```python
from build123d import *

# Parameters (mm, degrees)
BOSS_EXTRUDE1_DEPTH = 14
SKETCH2_R           = 2.5
SKETCH2_R_2         = 2.25
BOSS_EXTRUDE3_DEPTH = 1.5
SKETCH3_R           = 0.75
BOSS_EXTRUDE4_DEPTH = 8
BOSS_EXTRUDE5_DEPTH = 25.5
SKETCH8_R           = 0.75
BOSS_EXTRUDE7_DEPTH = 1
SKETCH9_R           = 0.75
BOSS_EXTRUDE8_DEPTH = 1


with BuildPart() as part:
    # Sketch1 → Boss-Extrude1 (new body)
    with BuildSketch(Plane.XY):
        with BuildLine():
            Line((1, 0), (23.320898327, 0))
            ThreePointArc((23.320898327, 0), (24.381558498, -0.439339828), (24.820898327, -1.5))
            Line((24.820898327, -1.5), (24.820898327, -11.016992716))
            ThreePointArc((24.820898327, -11.016992716), (24.381558498, -12.077652887), (23.320898327, -12.516992716))
            Line((23.320898327, -12.516992716), (1, -12.516992716))
            ThreePointArc((1, -12.516992716), (0.292893219, -12.224099497), (0, -11.516992716))
            Line((0, -11.516992716), (0, -1))
            ThreePointArc((0, -1), (0.292893219, -0.292893219), (1, 0))
        make_face()
    extrude(amount=BOSS_EXTRUDE1_DEPTH)

    # Sketch2 → Boss-Extrude3 (add)
    with BuildSketch(Plane(origin=(0, 0, 0), x_dir=(0, 0, -1), z_dir=(1, 0, 0))):
        with Locations((-7.367821443, -5.872283843)):
            Circle(SKETCH2_R)
        with Locations((-7.367821443, -5.872283843)):
            Circle(SKETCH2_R_2, mode=Mode.SUBTRACT)
    extrude(amount=-BOSS_EXTRUDE3_DEPTH)

    # Sketch3 → Boss-Extrude4 (add)
    with BuildSketch(Plane.ZY):
        with Locations(Location((7.367821443, -5.872283843, 0), (0, 0, 180))):
            Circle(SKETCH3_R)
    extrude(amount=BOSS_EXTRUDE4_DEPTH)

    # Sketch7 → Boss-Extrude5 (add)
    with BuildSketch(Plane(origin=(0, 0, 0), x_dir=(0, 0, -1), z_dir=(1, 0, 0))):
        with BuildLine():
            Line((-11.394447379, -3.62022901), (-3.393359944, -3.62022901))
            ThreePointArc((-3.393359944, -3.62022901), (-7.393903662, -9.38997212), (-11.394447379, -3.62022901))
        make_face()
    extrude(amount=BOSS_EXTRUDE5_DEPTH)

    # Sketch8 → Boss-Extrude7 (add)
    with BuildSketch(Plane(origin=(25.5, 0, 0), x_dir=(0, 0, -1), z_dir=(1, 0, 0))):
        with Locations((-7.348346706, -5.904616391)):
            Circle(SKETCH8_R)
    extrude(amount=-BOSS_EXTRUDE7_DEPTH)

    # Sketch9 → Boss-Extrude8 (add)
    with BuildSketch(Plane(origin=(25.5, 0, 0), x_dir=(0, 0, -1), z_dir=(1, 0, 0))):
        with Locations((-7.305909656, -5.926147043)):
            Circle(SKETCH9_R)
    extrude(amount=BOSS_EXTRUDE8_DEPTH)


solid = part.part
```
Design review of the part built by this model. Coordinates are the model's own, in mm. A direction names the side the tool comes from. Coordinates: 2 decimals unless noted, no trailing zeros. Write each loop counter-clockwise with the first axis right and the second up, starting at its lowest first coordinate (ties: lowest second). Pieces come first, ordered by that corner, then holes. Notation, with made-up numbers: M 35.5,-18.5 L 49.5,-18.5 A18 cw 49.5,8.5 Z; hole C 24,-5.5 d1. An arc over 180 degrees is marked long. Answer as a JSON object with one key per item and string values.
Item 1: Wall thickness on probe 1 along X at (y, z) = (-4.5, 9); probe 2 along X at (y, z) = (-2.75, 12.5); probe 3 along Y at (x, z) = (-1, 8.5): over which ranges is each line inside the solid? List them lowest first.
Outcome:
{"probe 1": "0 to 25.5", "probe 2": "0 to 24.82", "probe 3": "-8.1 to -7.82, -3.93 to -3.64"}
Item 2: Insertion check: pin 1 Ø6 at (y, z) = (-11, 5.5) entering from -X; pin 2 Ø0.7 at (x, z) = (25.5, 9) entering from +Y. Each pin has a flat end and moves straight along its axis. Give the tip position at first contact, or say it passes through.
Outcome:
{"pin 1": "x = -1.5", "pin 2": "y = -3.62"}
Item 3: Add section C-C, the plane x = -5. Give the boundary of the cut face in (y, z).
Outcome:
{"outline": "C -5.87,7.37 d1.5"}
Item 4: Add section D-D, the plane z = 6. Give the boundary of the cut face in (x, y).
Outcome:
{"outline": "M -1.5,-7.96 L 0,-7.96 L 0,-11.52 A1 ccw 1,-12.52 L 23.32,-12.52 A1.5 ccw 24.82,-11.02 L 24.82,-9.16 L 25.5,-9.16 L 25.5,-3.62 L 24.82,-3.62 L 24.82,-1.5 A1.5 ccw 23.32,0 L 1,0 A1 ccw 0,-1 L 0,-3.78 L -1.5,-3.78 L -1.5,-4.09 L 0,-4.09 L 0,-7.66 L -1.5,-7.66 Z"}
Item 5: Machinability: for faces 4 (the flat face through (13, -6, 14)), 5 (the flat face through (0, -5, 7)), 6 (the flat face through (24.821, -3, 7)), which of the approach directions +Z, -Z, +X, -X, +Y, -Y give a long, thin tool a straight path to every point of the face, cutting with its end or side? Answer none if there is none.
Outcome:
{"face 4": "+Z, +X, -X, +Y, -Y", "face 5": "-X", "face 6": "+X"}
Item 6: Draft analysis for pull direction Z (two halves, no side actions). For faces 1 (the flat face through (25.5, -5.8, 8.3)), 2 (the cylindrical face through (-0.74, -7.241, 9.153)), 3 (the cylindrical face through (-0.74, -5.762, 9.865)), state which applies: pulls with the +Z half, pulls with the -Z half, needs draft (parallel to the pull), parting line crosses it, or undercut.
Outcome:
{"face 1": "needs draft", "face 2": "undercut", "face 3": "parting line crosses it"}
Item 7: Add section A-A, the plane z = 1.25. Give the boundary of the cut face in (x, y), and give its area (3 significant figures).
Outcome:
{"outline": "M 0,-11.52 A1 ccw 1,-12.52 L 23.32,-12.52 A1.5 ccw 24.82,-11.02 L 24.82,-1.5 A1.5 ccw 23.32,0 L 1,0 A1 ccw 0,-1 Z", "area": "309 mm²"}
Item 8: Add section B-B, the plane y = -4.25. Give the boundary of the cut face in (x, z), and give its area (3 significant figures).
Outcome:
{"outline": "M -1.5,5.47 L 0,5.47 L 0,0 L 24.82,0 L 24.82,3.21 L 25.5,3.21 L 25.5,11.58 L 24.82,11.58 L 24.82,14 L 0,14 L 0,9.27 L -1.5,9.27 L -1.5,8.93 L 0,8.93 L 0,5.81 L -1.5,5.81 Z", "area": "354 mm²"}
